Can you work these out from the model? Positions are in its coordinate system, mm. Face numbers are marked on the shaded views. A direction names the side the tool comes from. Give positions to 0.01 mm unless a question says otherwise; leave off trailing zeros. Order: outer loops, then holes, each group sorted by start corner. A loop starts at its lowest first (then second) coordinate and runs counter-clockwise, first axis right, second up.
Item 1: I want a section at B-B, the plane y = 3. Write out the boundary of the cut face in (x, z).
Item 2: I want a section at C-C, the plane z = -14. Write out the boundary of the cut face in (x, y), then the cut area to 3 significant figures.
Item 3: If I drill on line 1 along Y through (x, z) = (36, 1.25); line 2 along Z through (x, y) = (-10, -6); line 3 along Y through (x, z) = (14, -11), over which ranges is the centre line in solid material (lowest first)?
Item 4: Which directions (+Z, -Z, +X, -X, +Y, -Y) give clear straight access to the entire face, cutting with the end or side of a thin tool? Please do the marked faces 1 and 2.
Item 5: I'm going to push flat-ended pins straight in: pin 1 Ø2 at (x, z) = (16.5, -12.5) entering from +Y; pin 2 Ø8 at (x, z) = (8.5, -10.5) entering from +Y; pin 3 Ø4 at (y, z) = (-18, -3.5) entering from +X. Where does each tip first touch, or does it pass through?
Item 6: I want a section at D-D, the plane y = 29.5. Write out the boundary of the cut face in (x, z).
Item 7: I want a section at A-A, the plane x = 32.5. Write out the boundary of the cut face in (y, z), then the cut area to 3 significant figures.
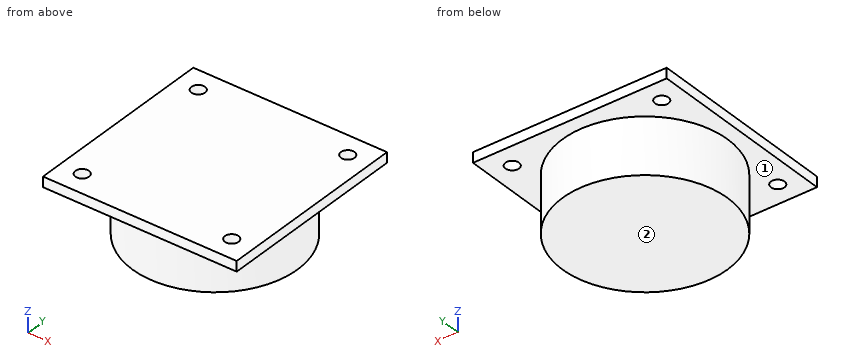
```python
from build123d import *

# Parameters (mm, degrees)
SKETCH2_W           = 57
SKETCH2_H           = 57
BOSS_EXTRUDE1_DEPTH = 3
SKETCH3_R           = 24.25
BOSS_EXTRUDE2_DEPTH = 16.5
SKETCH4_R           = 1.9939
CUT_EXTRUDE1_DEPTH  = 16.5


with BuildPart() as part:
    # Sketch2 → Boss-Extrude1 (new body)
    with BuildSketch(Plane.XY):
        with Locations((14.592, 4.446)):
            Rectangle(SKETCH2_W, SKETCH2_H)
    extrude(amount=BOSS_EXTRUDE1_DEPTH)

    # Sketch3 → Boss-Extrude2 (add)
    with BuildSketch(Plane(origin=(0, 0, 0), x_dir=(-1, 0, 0), z_dir=(0, 0, -1))):
        with Locations((-14.592, 4.446)):
            Circle(SKETCH3_R)
    extrude(amount=BOSS_EXTRUDE2_DEPTH)

    # Sketch4 → Cut-Extrude1 (cut)
    with BuildSketch(Plane.XY.offset(3)):
        with Locations((36.592, 26.446)):
            Circle(SKETCH4_R)
        with Locations((36.592, -17.554)):
            Circle(SKETCH4_R)
        with Locations((-7.408, -17.554)):
            Circle(SKETCH4_R)
        with Locations((-7.408, 26.446)):
            Circle(SKETCH4_R)
    extrude(amount=-CUT_EXTRUDE1_DEPTH, mode=Mode.SUBTRACT)


solid = part.part
```
Results list:
1. outline: (-13.91, 0) - (-9.61, 0) - (-9.61, -16.5) - (38.8, -16.5) - (38.8, 0) - (43.09, 0) - (43.09, 3) - (-13.91, 3) - close
2. outline: circle Ø48.5 at (14.59, 4.45)
2. area: 1,850 mm2
3. line 1: y = -24.05 to -19.46, -15.65 to 24.54, 28.35 to 32.95
3. line 2: z = 0 to 3
3. line 3: y = -19.8 to 28.69
4. face 1: -Z
4. face 2: -Z, +X, -X, +Y, -Y
5. pin 1: stops at y = 28.68
5. pin 2: stops at y = 28.61
5. pin 3: stops at x = 27.63
6. outline: (-13.91, 0) - (43.09, 0) - (43.09, 3) - (-13.91, 3) - close
7. outline: (-24.05, 0) - (-11.91, 0) - (-11.91, -16.5) - (20.8, -16.5) - (20.8, 0) - (32.95, 0) - (32.95, 3) - (-24.05, 3) - close
7. area: 711 mm2
